Autodesk Inventor part; units mm, degrees
ref_plane "YZ Plane" through (0, 0, 0) normal (1, 0, 0) x (0, 1, 0)
ref_plane "XZ Plane" through (0, 0, 0) normal (0, 1, 0) x (-1, 0, 0)
ref_plane "XY Plane" through (0, 0, 0) normal (0, 0, 1) x (1, 0, 0)
sketch "Sketch1" plane through (0, 0, 0) normal (0, 0, 1) x (1, 0, 0)
  line L0 (0, 0) -> (195.58, 0)
  line L1 (195.58, 0) -> (195.58, -88.9)
  line L2 (195.58, -88.9) -> (0, -88.9)
  line L3 (0, -88.9) -> (0, 0)
  dimension "d0" = 195.58
  dimension "d1" = 88.9
extrude "Extrusion1" add sketch "Sketch1" along normal blind 0.762
sketch "Sketch9" plane through (0, 0, 0.762) normal (0, 0, 1) x (1, 0, 0)
  line L0 (195.58, 0) -> (195.58, -88.9)
  line L1 (0, -88.9) -> (0, 0)
  line L2 (195.58, -88.9) -> (0, -88.9)
  line L3 (16.256, -54.61) -> (51.816, -54.61)
  line L4 (51.816, -54.61) -> (51.816, -73.66)
  line L5 (51.816, -73.66) -> (16.256, -73.66)
  line L6 (16.256, -73.66) -> (16.256, -54.61)
  line L7 (143.764, -54.61) -> (179.324, -54.61)
  line L8 (179.324, -54.61) -> (179.324, -73.66)
  line L9 (179.324, -73.66) -> (143.764, -73.66)
  line L10 (143.764, -73.66) -> (143.764, -54.61)
  line L11 (73.66, -50.8) -> (121.92, -50.8)
  line L12 (121.92, -50.8) -> (121.92, -78.74)
  line L13 (121.92, -78.74) -> (73.66, -78.74)
  line L14 (73.66, -78.74) -> (73.66, -50.8)
  dimension "d105" = 16.256
  dimension "d106" = 19.05
  dimension "d107" = 35.56
  dimension "d108" = 16.256
  dimension "d109" = 19.05
  dimension "d110" = 35.56
  dimension "d111" = 15.24
  dimension "d112" = 15.24
  dimension "d113" = 48.26
  dimension "d114" = 27.94
  dimension "d115" = 73.66
  dimension "d116" = 73.66
  dimension "d117" = 10.16
extrude "Extrusion4" cut sketch "Sketch9" against normal blind 25.4
sketch "Sketch10" plane through (0, 0, 0.762) normal (0, 0, 1) x (1, 0, 0)
  circle A0 centre (4.7625, -84.7725) radius 2.2479
  circle A1 centre (78.4225, -84.7725) radius 2.2479
  circle A2 centre (117.1575, -84.7725) radius 2.2479
  circle A3 centre (190.8175, -84.7725) radius 2.2479
  line L0 (195.58, -88.9) -> (0, -88.9)
  line L1 (0, -37.5396) -> (9.525, -37.5396)
  point P0 (4.7625, -33.02)
  point P1 (4.7625, -7.62)
  point P2 (78.4225, -7.62)
  point P3 (78.4225, -33.02)
  point P4 (117.1575, -33.02)
  point P5 (117.1575, -7.62)
  point P6 (190.8175, -33.02)
  point P7 (190.8175, -7.62)
  dimension "d127" = 81.28
  dimension "d128" = 55.88
  dimension "d129" = 55.88
  dimension "d130" = 81.28
  dimension "d131" = 81.28
  dimension "d132" = 55.88
  dimension "d133" = 55.88
  dimension "d134" = 81.28
hole "Hole5" at (190.8175, -84.7725, 0.762) at (117.1575, -84.7725, 0.762) at (78.4225, -84.7725, 0.762) at (4.7625, -84.7725, 0.762) at (4.7625, -7.62, 0.762) at (4.7625, -33.02, 0.762) at (78.4225, -33.02, 0.762) at (78.4225, -7.62, 0.762) at (117.1575, -7.62, 0.762) at (117.1575, -33.02, 0.762) at (190.8175, -33.02, 0.762) at (190.8175, -7.62, 0.762) direction (0, 0, -1) diameter 4.318 end through all
properties part number "ChassisFrontPlate" material "Steel"
Geometry: final body of the model. Coordinates: model frame, mm. Coordinates: 2 decimals unless noted, no trailing zeros. Order: outer loops, then holes, each group sorted by start corner. A loop starts at its lowest first (then second) coordinate and runs counter-clockwise, first axis right, second up.
(1) First-contact query: pin 1 (5.5 mm diameter, centred on x = 117.16, y = -7.62, fed in from -Z). Flat tip, straight axial feed; report the tip coordinate or a pass-through.
(2) Section query B-B (y = -77). Return the cut outline in (x, z), plus the area to 3 significant figures.
(3) Material intervals for probe 1 along X at (y, z) = (-33.02, 0.4); probe 2 along Y at (x, z) = (94, 0.15); probe 3 along X at (y, z) = (-54.5, 0.25), sorted ascending.
(4) Draft query along X for faces 1 (the face through (119.07, -85.77, 0.38)), 2 (the face through (96, -44, 0.762)). Return one class per face: pulls with the +X half, pulls with the -X half, needs draft (parallel to the pull), parting line crosses it, or undercut.
(5) Section query D-D (y = -67). Return the cut outline in (x, z), plus the area to 3 significant figures.
(6) Section query C-C (y = -33.02). Return the cut outline in (x, z).
(7) Section query A-A (x = 106.5). Return the cut outline in (y, z).
Solution:
1. pin 1: stops at z = 0
2. outline: (0, 0) - (73.66, 0) - (73.66, 0.76) - (0, 0.76) - close; (121.92, 0) - (195.58, 0) - (195.58, 0.76) - (121.92, 0.76) - close
2. area: 112 mm2
3. probe 1: x = 0 to 2.6, 6.92 to 76.26, 80.58 to 115, 119.32 to 188.66, 192.98 to 195.58
3. probe 2: y = -88.9 to -78.74, -50.8 to 0
3. probe 3: x = 0 to 73.66, 121.92 to 195.58
4. face 1: undercut
4. face 2: needs draft
5. outline: (0, 0) - (16.26, 0) - (16.26, 0.76) - (0, 0.76) - close; (51.82, 0) - (73.66, 0) - (73.66, 0.76) - (51.82, 0.76) - close; (121.92, 0) - (143.76, 0) - (143.76, 0.76) - (121.92, 0.76) - close; (179.32, 0) - (195.58, 0) - (195.58, 0.76) - (179.32, 0.76) - close
5. area: 58.1 mm2
6. outline: (0, 0) - (2.6, 0) - (2.6, 0.76) - (0, 0.76) - close; (6.92, 0) - (76.26, 0) - (76.26, 0.76) - (6.92, 0.76) - close; (80.58, 0) - (115, 0) - (115, 0.76) - (80.58, 0.76) - close; (119.32, 0) - (188.66, 0) - (188.66, 0.76) - (119.32, 0.76) - close; (192.98, 0) - (195.58, 0) - (195.58, 0.76) - (192.98, 0.76) - close
7. outline: (-88.9, 0) - (-78.74, 0) - (-78.74, 0.76) - (-88.9, 0.76) - close; (-50.8, 0) - (0, 0) - (0, 0.76) - (-50.8, 0.76) - close
